from build123d import *

# Parameters (mm, degrees)
BOSS_EXTRUDE1_DEPTH = 5
SKETCH3_W           = 42
SKETCH3_H           = 51
SKETCH3_W_2         = 35
SKETCH3_H_2         = 45.75
BOSS_EXTRUDE3_DEPTH = 25
SKETCH4_R           = 8.75
CUT_EXTRUDE2_DEPTH  = 5
CUT_EXTRUDE3_DEPTH  = 4
SKETCH7_W           = 6
SKETCH7_H           = 25
CUT_EXTRUDE4_DEPTH  = 4
SKETCH9_R           = 11
CUT_EXTRUDE5_DEPTH  = 4
SKETCH16_W          = 7
SKETCH16_H          = 30
BOSS_EXTRUDE5_DEPTH = 1.5
SKETCH17_W          = 7
SKETCH17_H          = 30
BOSS_EXTRUDE6_DEPTH = 1.5
SKETCH19_W          = 7
SKETCH19_H          = 30
BOSS_EXTRUDE7_DEPTH = 1.5
SKETCH18_R          = 1.4
CUT_EXTRUDE7_DEPTH  = 6
BOSS_EXTRUDE8_DEPTH = 30
SKETCH21_R          = 2.95
BOSS_EXTRUDE9_DEPTH = 4
SKETCH24_W          = 30
SKETCH24_H          = 20
CUT_EXTRUDE8_DEPTH  = 32
SKETCH25_R          = 2.5
SKETCH25_R_2        = 1.4
CUT_EXTRUDE9_DEPTH  = 5


with BuildPart() as part:
    # Sketch1 → Boss-Extrude1 (new body)
    with BuildSketch(Plane(origin=(0, 0, 0), x_dir=(1, 0, 0), z_dir=(0, 1, 0))):
        Polygon((21, 25.5), (-21, 25.5), (-21, -25.5), (-16, -25.5), (-11, -25.5), (11, -25.5), (16, -25.5), (21, -25.5), align=None)
    extrude(amount=BOSS_EXTRUDE1_DEPTH)

    # Sketch3 → Boss-Extrude3 (add)
    with BuildSketch(Plane(origin=(0, 5, 0), x_dir=(1, 0, 0), z_dir=(0, 1, 0))):
        Rectangle(SKETCH3_W, SKETCH3_H)
        Rectangle(SKETCH3_W_2, SKETCH3_H_2, mode=Mode.SUBTRACT)
    extrude(amount=BOSS_EXTRUDE3_DEPTH)

    # Sketch4 → Cut-Extrude2 (cut)
    with BuildSketch(Plane.ZY.offset(21)):
        with Locations((-12.5, 17.5)):
            Circle(SKETCH4_R)
    extrude(amount=-CUT_EXTRUDE2_DEPTH, mode=Mode.SUBTRACT)

    # Sketch6 → Cut-Extrude3 (cut)
    with BuildSketch(Plane(origin=(-17.5, 0, 0), x_dir=(0, 0, -1), z_dir=(1, 0, 0))):
        with BuildLine():
            Line((9.375, 17.5), (9.375, 30))
            Line((9.375, 30), (15.625, 30))
            Line((15.625, 30), (15.625, 17.5))
            ThreePointArc((15.625, 17.5), (12.5, 14.375), (9.375, 17.5))
        make_face()
    extrude(amount=-CUT_EXTRUDE3_DEPTH, mode=Mode.SUBTRACT)

    # Sketch7 → Cut-Extrude4 (cut)
    with BuildSketch(Plane.ZY.offset(21)):
        with Locations((2, 17.5)):
            Rectangle(SKETCH7_W, SKETCH7_H)
    extrude(amount=-CUT_EXTRUDE4_DEPTH, mode=Mode.SUBTRACT)

    # Sketch9 → Cut-Extrude5 (cut)
    with BuildSketch(Plane(origin=(21, 0, 0), x_dir=(0, 0, -1), z_dir=(1, 0, 0))):
        with Locations((12.5, 17.5)):
            Circle(SKETCH9_R)
    extrude(amount=-CUT_EXTRUDE5_DEPTH, mode=Mode.SUBTRACT)

    # Sketch16 → Boss-Extrude5 (add)
    with BuildSketch(Plane.ZY.offset(21)):
        with Locations((12, 15)):
            Rectangle(SKETCH16_W, SKETCH16_H)
    extrude(amount=BOSS_EXTRUDE5_DEPTH)

    # Sketch17 → Boss-Extrude6 (add)
    with BuildSketch(Plane(origin=(21, 0, 0), x_dir=(0, 0, -1), z_dir=(1, 0, 0))):
        with Locations((-12, 15)):
            Rectangle(SKETCH17_W, SKETCH17_H)
    extrude(amount=BOSS_EXTRUDE6_DEPTH)

    # Sketch19 → Boss-Extrude7 (add)
    with BuildSketch(Plane(origin=(0, 0, -25.5), x_dir=(-1, 0, 0), z_dir=(0, 0, -1))):
        with Locations((0, 15)):
            Rectangle(SKETCH19_W, SKETCH19_H)
    extrude(amount=BOSS_EXTRUDE7_DEPTH)

    # Sketch18 → Cut-Extrude7 (cut)
    with BuildSketch(Plane(origin=(0, 30, 0), x_dir=(1, 0, 0), z_dir=(0, 1, 0))):
        with Locations(Location((-20, -12, 0), (0, 0, 270))):
            Circle(SKETCH18_R)
        with Locations(Location((20, -12, 0), (0, 0, 90))):
            Circle(SKETCH18_R)
        with Locations(Location((0, 24.9375, 0), (0, 0, 270))):
            Circle(SKETCH18_R)
    extrude(amount=-CUT_EXTRUDE7_DEPTH, mode=Mode.SUBTRACT)

    # Sketch1_3 → Boss-Extrude8 (add)
    with BuildSketch(Plane(origin=(0, 0, 0), x_dir=(1, 0, 0), z_dir=(0, 1, 0))):
        Polygon((-11, -25.5), (-16, -25.5), (-16, -55.5), (-29, -55.5), (-29, -100.5), (-24, -100.5), (-24, -60.5), (24, -60.5), (24, -100.5), (29, -100.5), (29, -55.5), (16, -55.5), (16, -25.5), (11, -25.5), (11, -55.5), (-11, -55.5), align=None)
    extrude(amount=BOSS_EXTRUDE8_DEPTH)

    # Sketch21 → Boss-Extrude9 (add)
    with BuildSketch(Plane.ZY.offset(-24)):
        with Locations(Location((90.5, 15, 0), (0, 0, 180))):
            Circle(SKETCH21_R)
    extrude(amount=BOSS_EXTRUDE9_DEPTH)

    # Sketch24 → Cut-Extrude8 (cut)
    with BuildSketch(Plane.ZY.offset(16)):
        with Locations((40.5, 15)):
            Rectangle(SKETCH24_W, SKETCH24_H)
    extrude(amount=-CUT_EXTRUDE8_DEPTH, mode=Mode.SUBTRACT)

    # Sketch25 → Cut-Extrude9 (cut)
    with BuildSketch(Plane.ZY.offset(29)):
        with Locations((90.5, 15)):
            Circle(SKETCH25_R)
        with Locations((90.5, 22)):
            Circle(SKETCH25_R_2)
        with Locations((83.5, 15)):
            Circle(SKETCH25_R_2)
        with Locations(Location((90.5, 8, 0), (0, 0, 180))):
            Circle(SKETCH25_R_2)
        with Locations(Location((97.5, 15, 0), (0, 0, 180))):
            Circle(SKETCH25_R_2)
    extrude(amount=-CUT_EXTRUDE9_DEPTH, mode=Mode.SUBTRACT)


solid = part.part
For this review, take the finished solid that the model builds, in its own axes (mm). A direction names the side the tool comes from. Round coordinates to 2 decimals unless told otherwise and drop trailing zeros. Write each loop counter-clockwise with the first axis right and the second up, starting at its lowest first coordinate (ties: lowest second). Pieces come first, ordered by that corner, then holes. Notation, with made-up numbers: (42, -37.5) -> (92, -37.5) arc R11 cw to (92, -30.5) -> close; hole circle Ø2 at (88.25, 62). An arc over 180 degrees is marked (long way). Put each result on its own line as item: value.
Q1. Consider section A-A on x = -8. State the section outline as (y, z) points (3 decimals), and give its area (3 significant figures).
Determined:
outline: (0, -25.5) -> (30, -25.5) -> (30, -22.875) -> (5, -22.875) -> (5, 22.875) -> (30, 22.875) -> (30, 25.5) -> (0, 25.5) -> close; (0, 55.5) -> (30, 55.5) -> (30, 60.5) -> (0, 60.5) -> close
area: 536 mm^2
Q2. Clearance check with flat-ended pins moving along their axes: pin 1 Ø4 at (y, z) = (2.5, 33) entering from +X; pin 2 Ø9 at (x, y) = (-1, 20) entering from +Z; pin 3 Ø4 at (y, z) = (2.5, 41) entering from -X. State where each tip first meets the part, or that it passes through.
Determined:
pin 1: stops at x = 16
pin 2: stops at z = 60.5
pin 3: stops at x = -16
Q3. Consider section D-D on z = -12.5. State the section outline as (x, y) points.
Determined:
outline: (-21, 0) -> (21, 0) -> (21, 6.5) -> (17.5, 6.5) -> (17.5, 5) -> (-17.5, 5) -> (-17.5, 8.75) -> (-21, 8.75) -> close; (17.5, 28.5) -> (21, 28.5) -> (21, 30) -> (17.5, 30) -> close
Q4. Machinability: for faces 5 (the flat face through (20, 15, 91)), 6 (the flat face through (13, 5, 40)), 7 (the flat face through (-19, 28, -15.625)), 8 (the cylindrical face through (-27, 13, 89)), which of the approach directions +Z, -Z, +X, -X, +Y, -Y give a long, thin tool a straight path to every point of the face, cutting with its end or side? Answer none if there is none.
Determined:
face 5: +Z, +Y, -Y
face 6: +X, -X
face 7: -X, +Y
face 8: -X
Q5. To check wall thickness, follow L1, parallel to Z at x = -8.5, y = 18.5 (3 decimals); L2, parallel to X at y = 28.3, z = 12; L3, parallel to Z at x = -2, y = 19.25 (3 decimals). State the ranges of each line that lie inside material, in increasing order. Write a range as [from, to].
Determined:
L1: z = [-25.5, -22.875], [22.875, 25.5], [55.5, 60.5]
L2: x = [-22.5, -21.4], [-18.6, -17.5], [17.5, 18.6], [21.4, 22.5]
L3: z = [-27, -22.875], [22.875, 25.5], [55.5, 60.5]
Q6. Consider section B-B on z = 90.5. State the section outline as (x, y) points, and give its area (3 significant figures).
Determined:
outline: (-29, 0) -> (-24, 0) -> (-24, 6.6) -> (-29, 6.6) -> close; (-29, 9.4) -> (-24, 9.4) -> (-24, 12.5) -> (-29, 12.5) -> close; (-29, 17.5) -> (-24, 17.5) -> (-24, 20.6) -> (-29, 20.6) -> close; (-29, 23.4) -> (-24, 23.4) -> (-24, 30) -> (-29, 30) -> close; (20, 12.05) -> (24, 12.05) -> (24, 0) -> (29, 0) -> (29, 30) -> (24, 30) -> (24, 17.95) -> (20, 17.95) -> close
area: 271 mm^2
Q7. The part is to be moulded in two halves that separate along X. For faces 1 (the flat face through (0, 15, 25.5)), 2 (the flat face through (0, 24, -25)), 3 (the flat face through (-19, 28, -9.375)), 4 (the flat face through (16, 2, 41)), say which applies: released by +X, released by -X, zero draft, split by the parting line, or undercut.
Determined:
face 1: undercut
face 2: undercut
face 3: zero draft
face 4: released by +X
